```python
from build123d import *

# Parameters (mm, degrees)
F0_R     = 4
F1_DEPTH = 22
F0_R_2   = 5
F2_DEPTH = 15
F0_R_3   = 6
F3_DEPTH = 2
F4_D     = 3.4


with BuildPart() as f1:
    # F0 (on Top) → F1 (new body)
    with BuildSketch(Plane.XY):
        Circle(F0_R)
    extrude(amount=F1_DEPTH)

    # F0 (on Top) → F2 (join)
    with BuildSketch(Plane.XY):
        Circle(F0_R_2)
        Circle(F0_R, mode=Mode.SUBTRACT)
    extrude(amount=F2_DEPTH)

    # F0 (on Top) → F3 (join)
    with BuildSketch(Plane.XY):
        Circle(F0_R_3)
        Circle(F0_R_2, mode=Mode.SUBTRACT)
    extrude(amount=F3_DEPTH)

    # F4 (through all)
    with Locations(Plane(origin=(0, 0, 0), x_dir=(1, 0, 0), z_dir=(0, 0, -1))):
        with Locations((0, 0)):
            Hole(F4_D / 2)


solid = f1.part
```
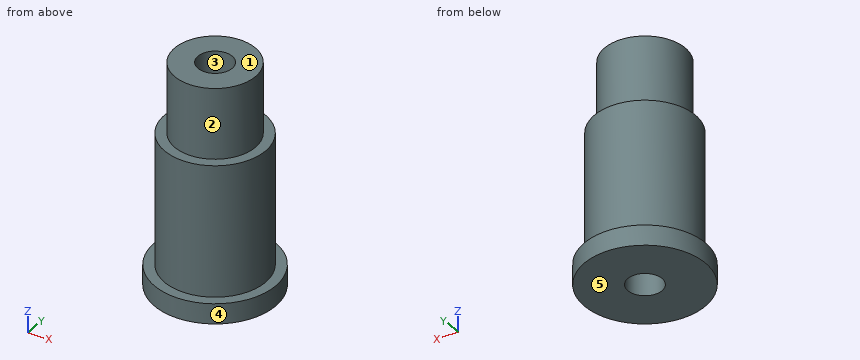
The listing builds one solid part. Answer for the finished solid, in the listing's coordinates (mm). Face numbers are marked on the shaded views. A direction names the side the tool comes from. Round coordinates to 2 decimals unless told otherwise and drop trailing zeros. Loops run counter-clockwise (first coordinate to the right, second up) from the corner with the lowest first, then second, coordinate; pieces in that order, holes last.
Q1. Which of the six approach directions +Z, -Z, +X, -X, +Y, -Y give full straight-line access (tool end or side, diameter ignored) to the marked faces 1 and 2?
Q2. Section D-D, the plane y = 3.5 is taken. Determine the outline of the cut face in (x, z), then the cut area to 3 significant figures.
Q3. Find the intervals of material crossed by line 1 (Y direction, x = 0, z = 14.5); line 2 (Y direction, x = 0, z = 15.25); line 3 (Z direction, x = -4, y = 2.5), in increasing order.
Q4. Section A-A, the plane x = 0 is taken. Determine the outline of the cut face in (y, z).
Q5. Section C-C, the plane z = 16.75 is taken. Determine the outline of the cut face in (x, y), then the cut area to 3 significant figures.
Q6. Given pin 1 Ø2 at (x, z) = (1.5, 17.5) entering from -Y; pin 2 Ø5 at (x, y) = (-3.5, 1) entering from -Z; pin 3 Ø6 at (x, z) = (3.5, 16.5) entering from +Y; pin 4 Ø6 at (y, z) = (4, 8.5) entering from +X, each flat-ended and moving along its own axis, determine where each tip first touches the part or whether it passes through.
Q7. For a pull along X with two mould halves and no side action, classify the marked faces 3, 4 and 5 as released by +X, released by -X, zero draft, split by the parting line, or undercut.
Completed:
1. face 1: +Z, +X, -X, +Y, -Y
1. face 2: +Z
2. outline: (-4.87, 0) - (4.87, 0) - (4.87, 2) - (3.57, 2) - (3.57, 15) - (1.94, 15) - (1.94, 22) - (-1.94, 22) - (-1.94, 15) - (-3.57, 15) - (-3.57, 2) - (-4.87, 2) - close
2. area: 139 mm2
3. line 1: y = -5 to -1.7, 1.7 to 5
3. line 2: y = -4 to -1.7, 1.7 to 4
3. line 3: z = 0 to 15
4. outline: (-6, 0) - (-1.7, 0) - (-1.7, 22) - (-4, 22) - (-4, 15) - (-5, 15) - (-5, 2) - (-6, 2) - close; (1.7, 0) - (6, 0) - (6, 2) - (5, 2) - (5, 15) - (4, 15) - (4, 22) - (1.7, 22) - close
5. outline: circle Ø8 at (0, 0); hole circle Ø3.4 at (0, 0)
5. area: 41.2 mm2
6. pin 1: stops at y = -3.97
6. pin 2: stops at z = 0
6. pin 3: stops at y = 4.92
6. pin 4: stops at x = 4.9
7. face 3: undercut
7. face 4: split by the parting line
7. face 5: zero draft
